Input: dimensioned drawing with shaded views. Units: mm. Origin: part minimum x, y, z. A direction names the side the tool comes from. Give positions to 0.01 mm unless a question says otherwise; leave off trailing zeros. Write each loop counter-clockwise with the first axis right and the second up, starting at its lowest first coordinate (ties: lowest second). Pieces come first, ordered by that corner, then holes.
Q1. Section A-A (x = 8). Return the cut outline in (y, z).
Q2. Section B-B (y = 46). Return the cut outline in (x, z).
Q3. Section C-C (z = 11). Return the cut outline in (x, y), plus the area to 3 significant figures.
Q4. Reachability of the marked faces 1, 2, 3 and 4 from +Z, -Z, +X, -X, +Y, -Y: full face, straight path, thin tool, end or side. Return the list, or none.
Q5. Section D-D (x = 43). Return the cut outline in (y, z), plus the area to 3 significant figures.
Q6. Line query: line 1 (Z direction, x = 6.5, y = 23.5); line 2 (Z direction, x = 43.5, y = 26); line 3 (Z direction, x = 13.5, y = 52). Output: solid intervals per line, ascending.
Q7. Pin query (flat end, axial travel): pin 1 Ø5 at (y, z) = (19, 24) entering from -X; pin 2 Ø11 at (y, z) = (21, 16) entering from +X; pin 3 Ø11 at (y, z) = (26, 44) entering from +X. Return the tip coordinate at first contact, or that it passes through.
Q8. Mould query, pull axis Z, two halves, no side actions, for the marked faces 5, 6 and 7. Classes: +Z half, -Z half, draft (parallel to the pull), parting line (faces both ways), or undercut.
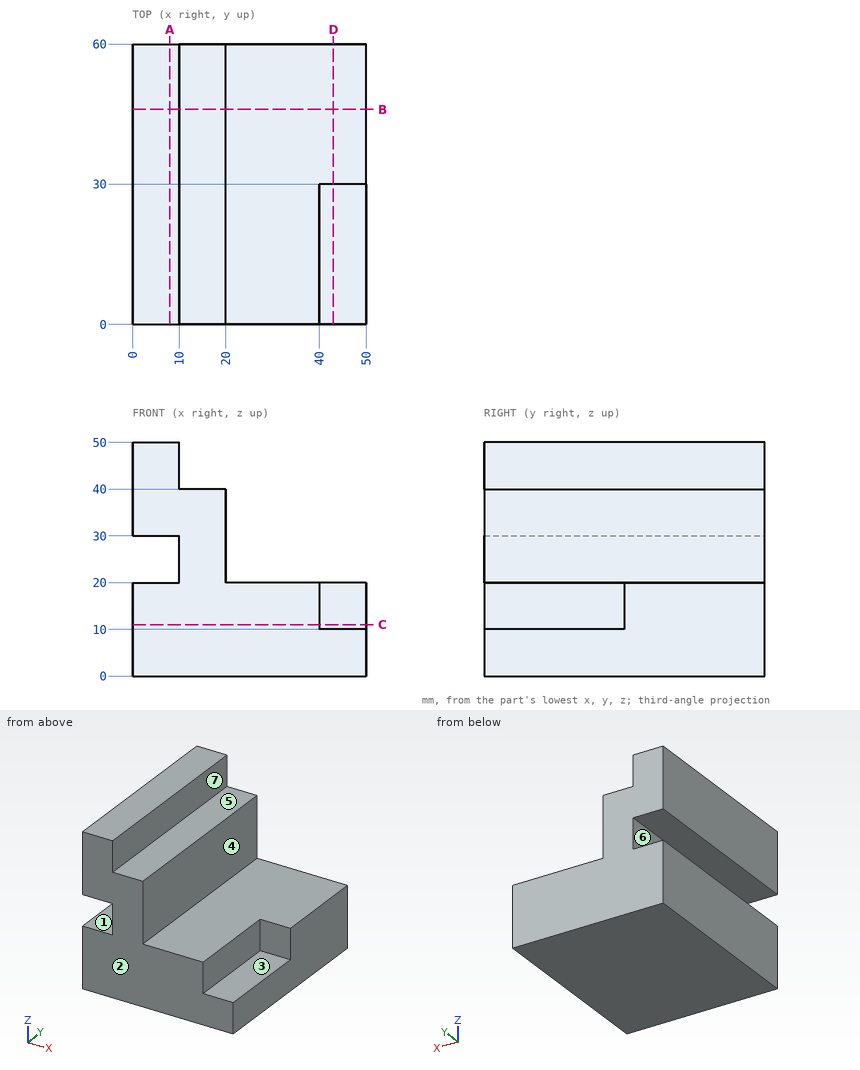
Computed:
1. outline: (0, 0) - (60, 0) - (60, 20) - (0, 20) - close; (0, 30) - (60, 30) - (60, 50) - (0, 50) - close
2. outline: (0, 0) - (50, 0) - (50, 20) - (20, 20) - (20, 40) - (10, 40) - (10, 50) - (0, 50) - (0, 30) - (10, 30) - (10, 20) - (0, 20) - close
3. outline: (0, 0) - (40, 0) - (40, 30) - (50, 30) - (50, 60) - (0, 60) - close
3. area: 2,700 mm2
4. face 1: -X, +Y, -Y
4. face 2: +Z, -Z, +X, -X, -Y
4. face 3: +Z, +X, -Y
4. face 4: +Z, +X, +Y, -Y
5. outline: (0, 0) - (60, 0) - (60, 20) - (30, 20) - (30, 10) - (0, 10) - close
5. area: 900 mm2
6. line 1: z = 0 to 20, 30 to 50
6. line 2: z = 0 to 10
6. line 3: z = 0 to 40
7. pin 1: stops at x = 10
7. pin 2: stops at x = 40
7. pin 3: stops at x = 20
8. face 5: +Z half
8. face 6: undercut
8. face 7: draft
